Work out the finished part from the listing and answer in its coordinate system (mm). Face numbers are marked on the shaded views. A direction names the side the tool comes from. Round coordinates to 2 decimals unless told otherwise and drop trailing zeros. Order: outer loops, then holes, each group sorted by start corner. A loop starts at its lowest first (then second) coordinate and runs counter-clockwise, first axis right, second up. Notation, with made-up numbers: (69.25, -21.5) -> (77.25, -21.5) arc R10 ccw to (77.25, -4.5) -> close; hole circle Ø10 at (16, 19). An arc over 180 degrees is marked (long way). Use a Markdown table: item, result. Add a question column.
Item 1: A cutting plane is placed at B-B, the plane z = 2.75. Determine the outline of the cut face in (x, y).
Item 2: A cutting plane is placed at D-D, the plane x = -20.5. Determine the outline of the cut face in (y, z), plus the area to 3 significant figures.
Item 3: A tool of negligible diameter and unlimited length cuts with its end or side. For the marked faces 4 and 5, from which of +Z, -Z, +X, -X, +Y, -Y can it reach the whole face along a straight path? Write none if from no direction.
Item 4: A cutting plane is placed at A-A, the plane y = -23.5. Determine the outline of the cut face in (x, z), plus the area to 3 significant figures.
Item 5: Find the intervals of material crossed by L1, parallel to Y at x = -45, z = 3.25; L2, parallel to X at y = -25.5, z = 7.25; L3, parallel to X at y = -21, z = 7.25, in increasing order. Write a range as [from, to].
Item 6: A cutting plane is placed at C-C, the plane y = -17.7. Determine the outline of the cut face in (x, z), plus the area to 3 significant figures.
Item 7: For a pull along X with two mould halves and no side action, classify the marked faces 1, 2 and 3 as +X half, -X half, draft (parallel to the pull), parting line (faces both ways), or undercut.
Item 8: Flat-ended cylindrical pins translate along their axes: P1, Ø4, axis at x = -16, z = 3.5, coming from the -Y side; P2, Ø2, axis at y = -15.5, z = 7.5, coming from the +X side; P3, Ø6, axis at x = -33, z = 3, coming from the +Y side. Find the tip coordinate at first contact, or state that the pin passes through.
from build123d import *

# Parameters (mm, degrees)
CROQUIS1_R              = 2.273640803
CROQUIS1_R_2            = 2.739354484
SALIENTE_EXTRUIR1_DEPTH = 10


with BuildPart() as part:
    # Croquis1 → Saliente-Extruir1 (new body)
    with BuildSketch(Plane.XY):
        with BuildLine():
            Line((-58.5, -33.5), (-58.5, -16.5))
            ThreePointArc((-58.5, -16.5), (-56.171439372, -10.87835735), (-50.549796722, -8.549796722))
            Line((-50.549796722, -8.549796722), (-40.505582208, -8.549796722))
            Line((-40.505582208, -8.549796722), (-8.795660821, -15.698566958))
            ThreePointArc((-8.795660821, -15.698566958), (-2.605899054, -24.392438678), (-10.567, -31.5))
            Line((-10.567, -31.5), (-18.5, -31.5))
            Line((-18.5, -31.5), (-18.5, -33.5))
            Line((-18.5, -33.5), (-58.5, -33.5))
        make_face()
        with Locations((-45.067, -17.7)):
            Circle(CROQUIS1_R, mode=Mode.SUBTRACT)
        with Locations((-10.567, -23.5)):
            Circle(CROQUIS1_R_2, mode=Mode.SUBTRACT)
    extrude(amount=SALIENTE_EXTRUIR1_DEPTH)


solid = part.part
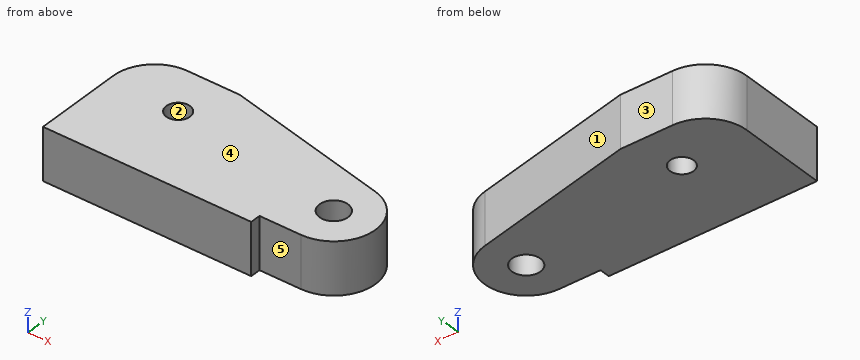
Reported:
| question | item | result |
|---|---|---|
| 1 | outline | (-58.5, -33.5) -> (-18.5, -33.5) -> (-18.5, -31.5) -> (-10.57, -31.5) arc R8 ccw to (-8.8, -15.7) -> (-40.51, -8.55) -> (-50.55, -8.55) arc R7.95 ccw to (-58.5, -16.5) -> close; hole circle Ø4.55 at (-45.07, -17.7); hole circle Ø5.48 at (-10.57, -23.5) |
| 2 | outline | (-33.5, 0) -> (-13.06, 0) -> (-13.06, 10) -> (-33.5, 10) -> close |
| 2 | area | 204 mm² |
| 3 | face 4 | +Z, +X, -X, +Y, -Y |
| 3 | face 5 | +Z, -Z, +X, -Y |
| 4 | outline | (-58.5, 0) -> (-13.31, 0) -> (-13.31, 10) -> (-58.5, 10) -> close; (-7.83, 0) -> (-2.56, 0) -> (-2.56, 10) -> (-7.83, 10) -> close |
| 4 | area | 505 mm² |
| 5 | L1 | [-33.5, -19.97], [-15.43, -8.55] |
| 5 | L2 | [-58.5, -12.44], [-8.7, -2.81] |
| 5 | L3 | [-58.5, -11.69], [-9.45, -2.96] |
| 6 | outline | (-58.5, 0) -> (-47.34, 0) -> (-47.34, 10) -> (-58.5, 10) -> close; (-42.79, 0) -> (-5.05, 0) -> (-5.05, 10) -> (-42.79, 10) -> close |
| 6 | area | 489 mm² |
| 7 | face 1 | +X half |
| 7 | face 2 | undercut |
| 7 | face 3 | draft |
| 8 | P1 | y = -31.5 |
| 8 | P2 | x = -6.69 |
| 8 | P3 | y = -9.57 |
